Input: part model. Units: mm. Frame: model coordinates. Face numbers are marked on the shaded views. Coordinates: 2 decimals unless noted, no trailing zeros. Write each loop counter-clockwise with the first axis right and the second up, starting at its lowest first coordinate (ties: lowest second). Pieces come first, ordered by that corner, then holes. Notation, with made-up numbers: (87.25, 48.25) - (120.25, 48.25) arc R26 ccw to (120.25, 64.25) - close; hole circle Ø7 at (39, 59.5). An arc over 180 degrees is marked (long way). Put each result on its own line as item: value. Start each with the question number.
1. Pin query (flat end, axial travel): pin 1 (1.5 mm diameter, centred on x = 7.5, z = 36, fed in from -Y); pin 2 (3 mm diameter, centred on y = 33, z = 34, fed in from -X); pin 3 (10 mm diameter, centred on x = -5.5, z = 40.5, fed in from +Y). Return the tip coordinate at first contact, or that it passes through.
2. Cut plane C-C, the plane z = 32. Return loops of the section in (x, y).
3. Cut plane A-A, the plane y = 0. Return loops of the section in (x, z).
4. Line query: line 1 (X direction, y = 0.5, z = 24); line 2 (X direction, y = -3, z = 16.5); line 3 (Y direction, x = -18.5, z = 27). Output: solid intervals per line, ascending.
5. Pull-direction query (Z, two-part tool) for the marked faces 1, 2 and 3; classes: released by +Z, released by -Z, zero draft, split by the parting line, or undercut.
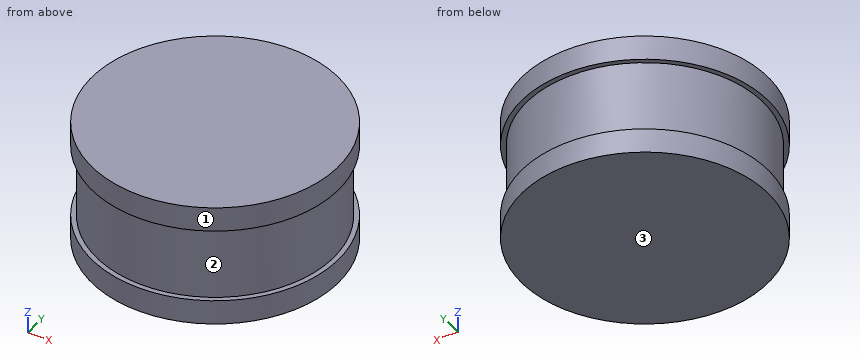
Solid Edge part; units mm, degrees
sketch "Sketch1" plane through (0, 0, 0) normal (0, 0, 1) x (1, 0, 0)
  circle A0 centre (0, 0) radius 48
extrude "Protrusion1" add sketch "Sketch1" along normal blind 50
sketch "Sketch2" plane through (0, 0, 0) normal (0, 0, 1) x (1, 0, 0)
  circle A0 centre (0, 0) radius 50
  circle A1 centre (0, 0) radius 48
extrude "ExtrudedProtrusion_2" add sketch "Sketch2" along normal blind 10
sketch "Sketch3" plane through (0, 0, 50) normal (0, 0, 1) x (1, 0, 0)
  circle A0 centre (0, 0) radius 50
extrude "ExtrudedProtrusion_4" add sketch "Sketch3" against normal blind 10
properties material "Aluminum, 1060"
Report:
1. pin 1: stops at y = -47.52
1. pin 2: stops at x = -36.22
1. pin 3: stops at y = 50
2. outline: circle Ø96 at (0, 0)
3. outline: (-50, 0) - (50, 0) - (50, 10) - (48, 10) - (48, 40) - (50, 40) - (50, 50) - (-50, 50) - (-50, 40) - (-48, 40) - (-48, 10) - (-50, 10) - close
4. line 1: x = -48 to 48
4. line 2: x = -47.91 to 47.91
4. line 3: y = -44.29 to 44.29
5. face 1: zero draft
5. face 2: undercut
5. face 3: released by -Z
